```python
from build123d import *

# Parameters (mm, degrees)
SKETCH1_W           = 48
SKETCH1_H           = 53
SKETCH1_R           = 1.9304
BOSS_EXTRUDE1_DEPTH = 10
SKETCH2_W           = 48
SKETCH2_H           = 5.616325
BOSS_EXTRUDE2_DEPTH = 33.1917878
SKETCH4_W           = 4
SKETCH4_H           = 10
BOSS_EXTRUDE4_DEPTH = 40
SKETCH5_W           = 48
SKETCH5_H           = 10.8609375
BOSS_EXTRUDE5_DEPTH = 23.1917878
SKETCH6_W           = 48
SKETCH6_H           = 5
BOSS_EXTRUDE6_DEPTH = 42.3
CUT_EXTRUDE1_REACH  = 78.862
SKETCH8_R           = 11.5
SKETCH9_R           = 1.9304
CUT_EXTRUDE2_DEPTH  = 88.252507127
CUT_EXTRUDE3_REACH  = 89.253
SKETCH10_W          = 3.15468
SKETCH10_H          = 6.8326
BOSS_EXTRUDE7_START = 8
SKETCH11_W          = 48
SKETCH11_H          = 42.3
SKETCH11_R          = 11.5
BOSS_EXTRUDE7_DEPTH = 8
SKETCH12_W          = 48
SKETCH12_H          = 42.3
BOSS_EXTRUDE8_DEPTH = 8
FILLET1_R           = 11
BOSS_EXTRUDE9_DEPTH = 3
CUT_EXTRUDE4_DEPTH  = 6
CUT_EXTRUDE5_DEPTH  = 90.10667764


with BuildPart() as part:
    # Sketch1 → Boss-Extrude1 (new body)
    with BuildSketch(Plane.XY):
        with Locations((24, 26.5)):
            Rectangle(SKETCH1_W, SKETCH1_H)
        with Locations((8.975, 38)):
            Circle(SKETCH1_R, mode=Mode.SUBTRACT)
        with Locations((38.975, 38)):
            Circle(SKETCH1_R, mode=Mode.SUBTRACT)
    extrude(amount=BOSS_EXTRUDE1_DEPTH)

    # Sketch2 → Boss-Extrude2 (add)
    with BuildSketch(Plane(origin=(0, 0, 0), x_dir=(-1, 0, 0), z_dir=(0, 0, -1))):
        with Locations((-24, -2.8081625)):
            Rectangle(SKETCH2_W, SKETCH2_H)
    extrude(amount=-BOSS_EXTRUDE2_DEPTH)

    # Sketch4 → Boss-Extrude4 (add)
    with BuildSketch(Plane.XY.offset(10)):
        with Locations((2, 48)):
            Rectangle(SKETCH4_W, SKETCH4_H)
        with Locations((46, 48)):
            Rectangle(SKETCH4_W, SKETCH4_H)
    extrude(amount=BOSS_EXTRUDE4_DEPTH)

    # Sketch5 → Boss-Extrude5 (add)
    with BuildSketch(Plane.XY.offset(10)):
        with Locations((24, 5.43046875)):
            Rectangle(SKETCH5_W, SKETCH5_H)
    extrude(amount=BOSS_EXTRUDE5_DEPTH)

    # Sketch6 → Boss-Extrude6 (add)
    with BuildSketch(Plane.XZ.offset(5.616325)):
        with Locations((24, 30.6917878)):
            Rectangle(SKETCH6_W, SKETCH6_H)
    extrude(amount=BOSS_EXTRUDE6_DEPTH)

    # Sketch8 → Cut-Extrude1 (cut, up to next)
    with BuildSketch(Plane(origin=(0, 0, 28.1917878), x_dir=(-1, 0, 0), z_dir=(0, 0, -1)), mode=Mode.PRIVATE) as cut_extrude1_sk1:
        with Locations((-24, -26.616325)):
            Circle(SKETCH8_R)
    cut_extrude1_tool1 = extrude(cut_extrude1_sk1.sketch, amount=-CUT_EXTRUDE1_REACH, mode=Mode.PRIVATE) & part.part
    add(cut_extrude1_tool1.solids().sort_by_distance((24, -26.616325, 28.191788))[0], mode=Mode.SUBTRACT)

    # Sketch9 → Cut-Extrude2 (cut, through all)
    with BuildSketch(Plane(origin=(48, 0, 0), x_dir=(0, 0, -1), z_dir=(1, 0, 0))):
        with Locations((-17, 48)):
            Circle(SKETCH9_R)
    extrude(amount=-CUT_EXTRUDE2_DEPTH, mode=Mode.SUBTRACT)

    # Sketch10 → Cut-Extrude3 (cut, up to next)
    with BuildSketch(Plane(origin=(0, 0, 0), x_dir=(-1, 0, 0), z_dir=(0, 0, -1)), mode=Mode.PRIVATE) as cut_extrude3_sk1:
        with Locations((-35.42266, 48)):
            Rectangle(SKETCH10_W, SKETCH10_H)
    cut_extrude3_tool1 = extrude(cut_extrude3_sk1.sketch, amount=-CUT_EXTRUDE3_REACH, mode=Mode.PRIVATE) & part.part
    # Sketch10 → Cut-Extrude3 (cut, up to next)
    with BuildSketch(Plane(origin=(0, 0, 0), x_dir=(-1, 0, 0), z_dir=(0, 0, -1)), mode=Mode.PRIVATE) as cut_extrude3_sk2:
        with Locations((-12.57734, 48)):
            Rectangle(SKETCH10_W, SKETCH10_H)
    cut_extrude3_tool2 = extrude(cut_extrude3_sk2.sketch, amount=-CUT_EXTRUDE3_REACH, mode=Mode.PRIVATE) & part.part
    add(cut_extrude3_tool1.solids().sort_by_distance((35.42266, 48, 0))[0], mode=Mode.SUBTRACT)
    add(cut_extrude3_tool2.solids().sort_by_distance((12.57734, 48, 0))[0], mode=Mode.SUBTRACT)

    # Sketch11 → Boss-Extrude7 (add)
    with BuildSketch(Plane(origin=(0, 0, 28.1917878), x_dir=(-1, 0, 0), z_dir=(0, 0, -1)).offset(BOSS_EXTRUDE7_START)):
        with Locations((-24, -26.766325)):
            Rectangle(SKETCH11_W, SKETCH11_H)
        with Locations((-24, -26.616325)):
            Circle(SKETCH11_R, mode=Mode.SUBTRACT)
    extrude(amount=-BOSS_EXTRUDE7_DEPTH)

    # Sketch12 → Boss-Extrude8 (add)
    with BuildSketch(Plane(origin=(0, 0, 20.1917878), x_dir=(-1, 0, 0), z_dir=(0, 0, -1))):
        with Locations((-24, -26.766325)):
            Rectangle(SKETCH12_W, SKETCH12_H)
    extrude(amount=BOSS_EXTRUDE8_DEPTH)

    # Fillet1
    fillet1_edges = [part.edges().sort_by_distance(p)[0] for p in [
        (24, -5.616325, 0),
    ]]
    fillet(fillet1_edges, radius=FILLET1_R)

    # Sketch13 → Boss-Extrude9 (add)
    with BuildSketch(Plane(origin=(0, 53, 0), x_dir=(1, 0, 0), z_dir=(0, 1, 0))):
        Polygon((0, 0), (0, -50), (4, -50), (4, -10), (44, -10), (44, -50), (48, -50), (48, 0), align=None)
    extrude(amount=BOSS_EXTRUDE9_DEPTH)

    # Sketch14 → Cut-Extrude4 (cut)
    with BuildSketch(Plane.XY.offset(10)):
        Polygon((8.975, 41.9594682), (5.545999953, 39.9797341), (5.545999953, 36.0202659), (8.975, 34.0405318), (12.404000047, 36.0202659), (12.404000047, 39.9797341), align=None)
        Polygon((38.975, 41.9594682), (35.545999953, 39.9797341), (35.545999953, 36.0202659), (38.975, 34.0405318), (42.404000047, 36.0202659), (42.404000047, 39.9797341), align=None)
    extrude(amount=-CUT_EXTRUDE4_DEPTH, mode=Mode.SUBTRACT)

    # Sketch15 → Cut-Extrude5 (cut, through all)
    with BuildSketch(Plane(origin=(48, 0, 0), x_dir=(0, 0, -1), z_dir=(1, 0, 0))):
        Polygon((-12.1917878, -5.616325), (-21.691694695, -47.916325), (-12.1917878, -47.916325), align=None)
    extrude(amount=-CUT_EXTRUDE5_DEPTH, mode=Mode.SUBTRACT)


solid = part.part
```
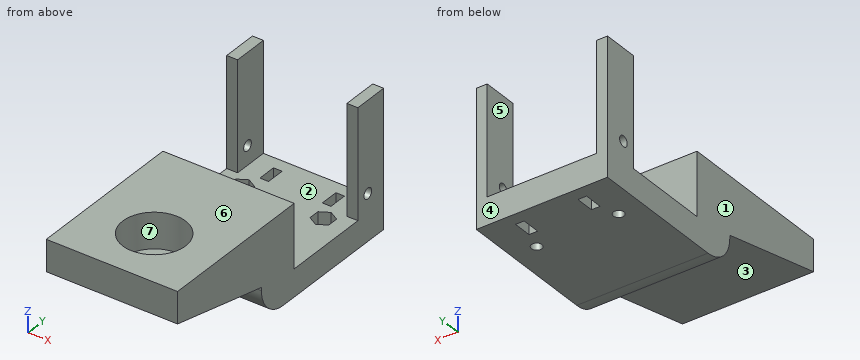
Input: part model. Units: mm. Frame: model coordinates. Face numbers are marked on the shaded views. A direction names the side the tool comes from. Round coordinates to 2 decimals unless told otherwise and drop trailing zeros. Order: outer loops, then holes, each group sorted by start corner. A loop starts at its lowest first (then second) coordinate and runs counter-clockwise, first axis right, second up. Notation, with made-up numbers: (-38, 22.25) - (-32, 22.25) arc R31 ccw to (-32, 56.25) - close; hole circle Ø9 at (-19.5, 18.5). An arc over 180 degrees is marked (long way). One line per question, with ' | ' between items. Start each with the question number.
1) Cut plane B-B, the plane z = 29.5. Return the cut outline in (x, y), then the cut area to 3 significant figures.
2) Pull-direction query (Y, two-part tool) for the marked faces 1, 2, 3 and 4; classes: +Y half, -Y half, draft (parallel to the pull), parting line (faces both ways), or undercut.
3) Contact query for flat-ended pins moving along their axis: P1, Ø12, axis at x = 35.5, z = 37.5, coming from the +Y side; P2, Ø10, axis at y = 34, z = 19, coming from the -X side; P3, Ø3.5, axis at x = 35.5, z = 6.5, coming from the -Y side; P4, Ø1, axis at x = 17.5, z = 6.5, coming from the -Y side. Output: stop coordinate, or through.
4) Set-up query: the marked faces 5, 6 and 7. Return all of +Z, -Z, +X, -X, +Y, -Y with unobstructed straight access to the full face (end or side cutting, diameter ignored); none if empty.
5) Cut plane D-D, the plane z = 36. Return the cut outline in (x, y).
6) Cut plane C-C, the plane x = 24. Return the cut outline in (y, z), then the cut area to 3 significant figures.
7) Ray query, probe 1 along X at (y, z) = (38, 2.4); probe 2 along X at (y, z) = (51, 16); probe 3 along Y at (x, z) = (24, 26). Return the intervals inside material, ascending.
8) Cut plane A-A, the plane y = 38. Return the cut outline in (x, z), then the cut area to 3 significant figures.
Worked out:
1) outline: (0, -47.92) - (48, -47.92) - (48, 10.86) - (0, 10.86) - close; (0, 43) - (4, 43) - (4, 56) - (0, 56) - close; (44, 43) - (48, 43) - (48, 56) - (44, 56) - close; hole circle Ø23 at (24, -26.62) | area: 2,510 mm^2
2) face 1: draft | face 2: undercut | face 3: -Y half | face 4: +Y half
3) P1: stops at y = 10.86 | P2: passes through | P3: stops at y = -5.27 | P4: stops at y = -4.86
4) face 5: +Z, +Y | face 6: +Z, +X, -X, -Y | face 7: +Z
5) outline: (0, 43) - (4, 43) - (4, 56) - (0, 56) - close; (44, 43) - (48, 43) - (48, 56) - (44, 56) - close
6) outline: (-47.92, 21.69) - (-5.62, 12.19) - (-5.62, 11) arc R11 ccw to (5.38, 0) - (56, 0) - (56, 10) - (10.86, 10) - (10.86, 33.19) - (-15.12, 33.19) - (-15.12, 20.19) - (-38.12, 20.19) - (-38.12, 33.19) - (-47.92, 33.19) - close | area: 1,360 mm^2
7) probe 1: x = 0 to 7.04, 10.91 to 37.04, 40.91 to 48 | probe 2: x = 0 to 4, 44 to 48 | probe 3: y = -47.92 to -38.12, -15.12 to 10.86
8) outline: (0, 0) - (7.04, 0) - (7.04, 4) - (5.55, 4) - (5.55, 10) - (0, 10) - close; (10.91, 0) - (37.04, 0) - (37.04, 4) - (35.55, 4) - (35.55, 10) - (12.4, 10) - (12.4, 4) - (10.91, 4) - close; (40.91, 0) - (48, 0) - (48, 10) - (42.4, 10) - (42.4, 4) - (40.91, 4) - close | area: 367 mm^2
